Geometry: final body of the model. Coordinates: model frame, mm. A direction names the side the tool comes from. Round coordinates to 2 decimals unless told otherwise and drop trailing zeros. Loops run counter-clockwise (first coordinate to the right, second up) from the corner with the lowest first, then second, coordinate; pieces in that order, holes last. Notation, with made-up numbers: (76.5, 18.5) - (104.5, 18.5) arc R21 ccw to (104.5, 23.5) - close; hole circle Ø7 at (-21.75, 88). An arc over 180 degrees is marked (long way). Answer as a JSON object with one key per item and string values. Group by question number.
Item 1: Reachability of faces 1 (the face through (26, 25.9, 1)), 2 (the face through (26, -25.9, 1)), 3 (the face through (0, -27.9, -1)), 4 (the face through (-26, -25.9, 1)) from +Z, -Z, +X, -X, +Y, -Y: full face, straight path, thin tool, end or side. Return the list, or none.
Item 2: Section A-A (z = -2.25). Return the cut outline in (x, y), plus the area to 3 significant figures.
Item 3: Section D-D (x = 14). Return the cut outline in (y, z).
Item 4: Draft query along Y for faces 5 (the face through (0, -25.9, -2)), 6 (the face through (0, 25.9, -2)), 7 (the face through (10, 27, -2)), 8 (the face through (-26, 25.9, 1)). Return one class per face: released by +Y, released by -Y, zero draft, split by the parting line, or undercut.
Item 5: First-contact query: pin 1 (2 mm diameter, centred on x = 30.5, z = 1, fed in from +Y); pin 2 (1 mm diameter, centred on x = 0, z = -4, fed in from +Y); pin 3 (1.4 mm diameter, centred on y = -28, z = -2, fed in from +X). Flat tips, straight axial feed; report the tip coordinate or a pass-through.
Item 6: Section C-C (y = -14). Return the cut outline in (x, z).
Item 7: Section B-B (x = -7.5). Return the cut outline in (y, z), plus the area to 3 significant figures.
Item 8: Line query: line 1 (Y direction, x = -7.5, z = -2.5); line 2 (Z direction, x = -37.5, y = -15); line 3 (Y direction, x = -6, z = 1.5). Output: solid intervals per line, ascending.
Autodesk Fusion 360 part; units mm, degrees
sketch "Boceto1" plane through (0, 0, 0) normal (0, 0, 1) x (1, 0, 0)
  line L0 (41.9, 25.9) -> (-41.9, 25.9)
  line L1 (-41.9, 25.9) -> (-41.9, -25.9)
  line L2 (-41.9, -25.9) -> (41.9, -25.9)
  line L3 (41.9, -25.9) -> (41.9, 25.9)
  line L4 (41.9, 25.9) -> (-41.9, -25.9) construction
  line L5 (-41.9, 25.9) -> (41.9, -25.9) construction
  dimension "d1" = 83.8
  dimension "d2" = 51.8
extrude "Extruir1" add sketch "Boceto1" along normal blind 2
sketch "Boceto4" plane through (0, 0, 0) normal (1, 0, 0) x (0, 1, 0)
  line L0 (25.9, 2) -> (27.9, 2)
  line L1 (27.9, 2) -> (27.9, -5.3)
  line L2 (27.9, -5.3) -> (25.9, -5.3)
  line L3 (25.9, -5.3) -> (25.9, 2)
  line L4 (25.9, -5.3) -> (24.8996, -3.8)
  line L5 (25.9, -5.3) -> (27.703, -5.3) construction
  line L6 (24.8996, -3.8) -> (25.9, -3.8)
  line L7 (27.9, -5.3) -> (29.9, -5.3)
  line L8 (27.9, -5.3) -> (27.9, -3.3)
  line L9 (27.9, -3.3) -> (29.9, -5.3)
  line L10 (0, 7.5) -> (0, -4)
  line L11 (-25.9, -5.3) -> (-25.9, 2)
  line L12 (-25.9, 2) -> (-27.9, 2)
  line L13 (-27.9, 2) -> (-27.9, -5.3)
  line L14 (-27.9, -5.3) -> (-29.9, -5.3)
  line L15 (-27.9, -5.3) -> (-27.9, -3.3)
  line L16 (-27.9, -3.3) -> (-29.9, -5.3)
  line L17 (-24.8996, -3.8) -> (-25.9, -3.8)
  line L18 (-25.9, -5.3) -> (-24.8996, -3.8)
  line L19 (-25.9, -5.3) -> (-27.703, -5.3) construction
  line L20 (-27.9, -5.3) -> (-25.9, -5.3)
  dimension "d20" = 2
  dimension "d21" = 7.3
  dimension "d29" = 1.0004
  dimension "d30" = 1.803
  dimension "d31" = 2
  dimension "d32" = 2
extrude "Extruir5" add sketch "Boceto4" along normal mid plane 20
fillet "Empalme1" radius 0.25 2 edges at (0, 24.8996, -3.8) (0, -24.8996, -3.8)
equation "d21 = 2 mm + 5.3 mm"
Values:
{
 "1": {"face 1": "+Z, -Z, +X, +Y", "face 2": "+Z, -Z, +X, -Y", "face 3": "+Z, +X, -X, -Y", "face 4": "+Z, -Z, -X, -Y"},
 "2": {"outline": "(-10, -27.9) - (10, -27.9) - (10, -25.9) - (-10, -25.9) - close; (-10, 25.9) - (10, 25.9) - (10, 27.9) - (-10, 27.9) - close", "area": "80.0 mm^2"},
 "3": {"outline": "(-25.9, 0) - (25.9, 0) - (25.9, 2) - (-25.9, 2) - close"},
 "4": {"face 5": "undercut", "face 6": "undercut", "face 7": "zero draft", "face 8": "released by +Y"},
 "5": {"pin 1": "stops at y = 25.9", "pin 2": "stops at y = 29.1", "pin 3": "stops at x = 10"},
 "6": {"outline": "(-41.9, 0) - (41.9, 0) - (41.9, 2) - (-41.9, 2) - close"},
 "7": {"outline": "(-29.9, -5.3) - (-25.9, -5.3) - (-25.16, -4.19) arc R0.25 ccw to (-25.37, -3.8) - (-25.9, -3.8) - (-25.9, 0) - (25.9, 0) - (25.9, -3.8) - (25.37, -3.8) arc R0.25 ccw to (25.16, -4.19) - (25.9, -5.3) - (29.9, -5.3) - (27.9, -3.3) - (27.9, 2) - (-27.9, 2) - (-27.9, -3.3) - close", "area": "138 mm^2"},
 "8": {"line 1": "y = -27.9 to -25.9, 25.9 to 27.9", "line 2": "z = 0 to 2", "line 3": "y = -27.9 to 27.9"}
}
